Read the model definition and answer for the solid it produces. Units are mm, in the model's axes. Face numbers are marked on the shaded views. A direction names the side the tool comes from. Give positions to 0.01 mm unless a question says otherwise; leave off trailing zeros. Order: outer loops, then holes, each group sorted by start corner. A loop starts at its lowest first (then second) coordinate and runs counter-clockwise, first axis right, second up.
Item 1: Which of the six approach directions +Z, -Z, +X, -X, +Y, -Y give full straight-line access (tool end or side, diameter ignored) to the marked faces 1, 2, 3, 4 and 5?
Item 2: Given pin 1 Ø8 at (x, y) = (0, 8.5) entering from -Z; pin 2 Ø3 at (y, z) = (2, -9.5) entering from +X; pin 3 Ø12 at (y, z) = (2.5, 7.5) entering from +X; pin 4 Ø4 at (x, z) = (3.175, 6.35) entering from -Y, each flat-ended and moving along its own axis, determine where each tip first touches the part or whether it passes through.
Item 3: A cutting plane is placed at D-D (y = 9.75). Write down the section's boundary in (x, z) (3 decimals).
Item 4: Find the intervals of material crossed by line 1 along X through (y, z) = (8.75, 0); line 2 along X through (y, z) = (10.75, 0); line 3 along Y through (x, z) = (0, -5), in increasing order.
Item 5: The mould has two halves that part along Z. Classify the marked faces 6, 7 and 8: +Z half, -Z half, draft (parallel to the pull), parting line (faces both ways), or undercut.
Item 6: A cutting plane is placed at A-A (z = 0). State how many separate pieces and enclosed holes the cut face has, plus the area to 3 significant figures.
from build123d import *

# Parameters (mm, degrees)
SKETCH1_R               = 11.43
BOSS_EXTRUDE1_DEPTH     = 13.97
CUT_EXTRUDE1_DEPTH      = 5.08
CUT_EXTRUDE2_DEPTH      = 22.364706878
CUT_EXTRUDE2_DEPTH_BACK = 22.364706878
SKETCH3_R               = 2.286
FILLET1_R               = 1.27
SKETCH4_R               = 17.78
SKETCH4_R_2             = 11.43
BOSS_EXTRUDE2_DEPTH     = 6.35
CUT_EXTRUDE3_DEPTH      = 38.588567411
CUT_EXTRUDE3_DEPTH_BACK = 4.826
SKETCH5_R               = 4.064
SKETCH7_R               = 1.778
CUT_EXTRUDE4_DEPTH      = 29.764869198
CHAMFER1_SIZE           = 5.08
FILLET2_R               = 2.54
SKETCH9_R               = 2.032
CUT_EXTRUDE5_DEPTH      = 10.16


with BuildPart() as part:
    # Sketch1 → Boss-Extrude1 (new, symmetric)
    with BuildSketch(Plane(origin=(0, 0, 0), x_dir=(1, 0, 0), z_dir=(0, 1, 0))):
        with Locations(Location((0, 0, 0), (0, 0, 270))):
            Circle(SKETCH1_R)
    extrude(amount=BOSS_EXTRUDE1_DEPTH, both=True)

    # Sketch2 → Cut-Extrude1 (cut, symmetric)
    with BuildSketch(Plane(origin=(0, 0, 0), x_dir=(1, 0, 0), z_dir=(0, 1, 0))):
        with BuildLine():
            Line((10.980176456, 3.175), (0.790573729, 3.175))
            ThreePointArc((0.790573729, 3.175), (1.644174222, 7.956847789), (-1.908379573, 11.269560213))
            ThreePointArc((-1.908379573, 11.269560213), (-9.679362018, 6.079050167), (-10.980176456, -3.175))
            Line((-10.980176456, -3.175), (-0.790573729, -3.175))
            ThreePointArc((-0.790573729, -3.175), (-1.644174222, -7.956847789), (1.908379573, -11.269560213))
            ThreePointArc((1.908379573, -11.269560213), (8.730912854, -7.376724255), (11.43, 0))
            ThreePointArc((11.43, 0), (11.316985396, 1.603353222), (10.980176456, 3.175))
        make_face()
    extrude(amount=CUT_EXTRUDE1_DEPTH, both=True, mode=Mode.SUBTRACT)

    # Sketch3 → Cut-Extrude2 (cut, two sides: drawn at the far end of the back side and taken through both)
    with BuildSketch(Plane(origin=(0, 0, 0), x_dir=(1, 0, 0), z_dir=(0, 1, 0)).offset(-CUT_EXTRUDE2_DEPTH_BACK)):
        with Locations(Location((-3.175, 6.35, 0), (0, 0, 270))):
            Circle(SKETCH3_R)
        with Locations(Location((3.175, -6.35, 0), (0, 0, 270))):
            Circle(SKETCH3_R)
    extrude(amount=CUT_EXTRUDE2_DEPTH + CUT_EXTRUDE2_DEPTH_BACK, mode=Mode.SUBTRACT)

    # Fillet1
    # the kernel refuses this fillet: 1.27 mm, written as the material it takes off along each edge
    with BuildSketch(Plane(origin=(-0.790573729, 5.08, 3.175), x_dir=(-0.4705483235385416, 0, 0.8823742262867087), z_dir=(0, -1, 0))) as fillet1_piece_1:
        with BuildLine():
            CenterArc((2.104974221, 1.248277745), FILLET1_R, 151.930104711, 107.457603124)
            Line((0.984358954, 1.845874115), (0, 0))
            ThreePointArc((0, 0), (0.935544098, 0.086889022), (1.871088197, 0))
        make_face()
    extrude(amount=10.16, mode=Mode.SUBTRACT)
    with BuildSketch(Plane(origin=(-10.980176456, 5.08, 3.175), x_dir=(0.35895527903729396, 0, 0.9333547598053263), z_dir=(0, -1, 0))) as fillet1_piece_2:
        with BuildLine():
            CenterArc((1.847316222, -1.265342552), FILLET1_R, 85.09157022, 115.944479772)
            Line((0.661955677, -1.721215757), (0, 0))
            ThreePointArc((0, 0), (0.977990941, 0.041917031), (1.955981882, 0))
        make_face()
    extrude(amount=10.16, mode=Mode.SUBTRACT)
    with BuildSketch(Plane(origin=(-1.908379573, -5.08, -11.269560213), x_dir=(0.9998377506147018, 0, 0.018013118712026065), z_dir=(0, 1, 0))) as fillet1_piece_3:
        with BuildLine():
            CenterArc((3.987576413, -1.248150652), FILLET1_R, 79.35661856, 136.209501667)
            ThreePointArc((2.954501471, -1.986836082), (1.657014707, -0.726102119), (0, 0))
            ThreePointArc((0, 0), (2.111069866, 0.196644134), (4.222139731, 0))
        make_face()
    extrude(amount=10.16, mode=Mode.SUBTRACT)
    with BuildSketch(Plane(origin=(0.790573729, -5.08, -3.175), x_dir=(1, 0, 0), z_dir=(0, 1, 0))) as fillet1_piece_4:
        with BuildLine():
            CenterArc((2.0919402, 1.27), FILLET1_R, 162.542396876, 107.457603124)
            ThreePointArc((0.880437414, 1.651), (0.516887341, 0.784614516), (0, 0))
            Line((0, 0), (2.0919402, 0))
        make_face()
    extrude(amount=10.16, mode=Mode.SUBTRACT)
    with BuildSketch(Plane(origin=(10.980176456, -5.08, -3.175), x_dir=(-0.3589552790375579, 0, -0.9333547598052248), z_dir=(0, 1, 0))) as fillet1_piece_5:
        with BuildLine():
            CenterArc((1.847316222, 1.265342552), FILLET1_R, 158.963950007, 115.944479772)
            Line((0.661955677, 1.721215757), (0, 0))
            ThreePointArc((0, 0), (0.977990941, -0.041917031), (1.955981882, 0))
        make_face()
    extrude(amount=10.16, mode=Mode.SUBTRACT)
    with BuildSketch(Plane(origin=(1.908379573, 5.08, 11.269560213), x_dir=(-0.9998377506147016, 0, -0.018013118712031834), z_dir=(0, -1, 0))) as fillet1_piece_6:
        with BuildLine():
            CenterArc((3.987576413, 1.248150652), FILLET1_R, 144.433879773, 136.209501667)
            ThreePointArc((2.954501471, 1.986836082), (1.657014707, 0.726102119), (0, 0))
            ThreePointArc((0, 0), (2.111069866, -0.196644134), (4.222139731, 0))
        make_face()
    extrude(amount=10.16, mode=Mode.SUBTRACT)

    # Sketch4 → Boss-Extrude2 (add)
    with BuildSketch(Plane(origin=(0, 13.97, 0), x_dir=(1, 0, 0), z_dir=(0, 1, 0))):
        with Locations(Location((0, 0, 0), (0, 0, 270))):
            Circle(SKETCH4_R)
        with Locations(Location((0, 0, 0), (0, 0, 270))):
            Circle(SKETCH4_R_2, mode=Mode.SUBTRACT)
    boss_extrude2 = extrude(amount=-BOSS_EXTRUDE2_DEPTH)

    # Mirror1: Boss-Extrude2 across plane
    add(boss_extrude2.mirror(Plane.ZX))

    # Sketch5 → Cut-Extrude3 (cut, two sides: drawn at the far end of the back side and taken through both)
    with BuildSketch(Plane(origin=(0, 13.97, 0), x_dir=(1, 0, 0), z_dir=(0, 1, 0)).offset(-CUT_EXTRUDE3_DEPTH_BACK)):
        with Locations(Location((-3.175, 6.35, 0), (0, 0, 90))):
            Circle(SKETCH5_R)
        with Locations(Location((3.175, -6.35, 0), (0, 0, 90))):
            Circle(SKETCH5_R)
    extrude(amount=CUT_EXTRUDE3_DEPTH + CUT_EXTRUDE3_DEPTH_BACK, mode=Mode.SUBTRACT)

    # Sketch7 → Cut-Extrude4 (cut, through all)
    with BuildSketch(Plane(origin=(0, 0, 0), x_dir=(1, 0, 0), z_dir=(0, 1, 0))):
        with Locations(Location((-4.064, 0, 0), (0, 0, 270))):
            Circle(SKETCH7_R)
        with Locations(Location((4.064, 0, 0), (0, 0, 90))):
            Circle(SKETCH7_R)
    extrude(amount=CUT_EXTRUDE4_DEPTH, mode=Mode.SUBTRACT)

    # Chamfer1
    chamfer1_edges = [part.edges().sort_by_distance(p)[0] for p in [
        (0, 7.62, -17.78),
        (0, -7.62, -17.78),
    ]]
    chamfer(chamfer1_edges, length=CHAMFER1_SIZE)

    # Fillet2
    # the kernel refuses this fillet: 2.54 mm, written as the material it adds along each edge
    with BuildSketch(Plane(origin=(0, 7.62, 0), x_dir=(0, 0, 1), z_dir=(-1, 0, 0))) as fillet2_piece_1:
        with BuildLine():
            CenterArc((13.97, -2.199704526), FILLET2_R, 120, 60)
            Line((12.7, 0), (12.6746, 0.043994091))
            ThreePointArc((12.6746, 0.043994091), (12.065, 0.0508), (11.43, 0.0508))
            Line((11.43, 0.0508), (11.3792, 0))
            Line((11.3792, 0), (11.3792, -2.199704526))
            Line((11.3792, -2.199704526), (11.43, -2.199704526))
        make_face()
    revolve(axis=Axis((0, 7.62, 0), (0, 1, 0)))
    with BuildSketch(Plane(origin=(0, -7.62, 0), x_dir=(0, 0, 1), z_dir=(-1, 0, 0))) as fillet2_piece_2:
        with BuildLine():
            CenterArc((13.97, 2.199704526), FILLET2_R, 180, 60)
            Line((11.43, 2.199704526), (11.3792, 2.199704526))
            Line((11.3792, 2.199704526), (11.3792, 0))
            Line((11.3792, 0), (11.43, -0.0508))
            ThreePointArc((11.43, -0.0508), (12.065, -0.0508), (12.6746, -0.043994091))
            Line((12.6746, -0.043994091), (12.7, 0))
        make_face()
    revolve(axis=Axis((0, -7.62, 0), (0, 1, 0)))

    # Sketch9 → Cut-Extrude5 (cut)
    with BuildSketch(Plane.XZ.offset(13.97)):
        with Locations(Location((0, 0, 0), (0, 0, 270))):
            Circle(SKETCH9_R)
    extrude(amount=-CUT_EXTRUDE5_DEPTH, mode=Mode.SUBTRACT)


solid = part.part
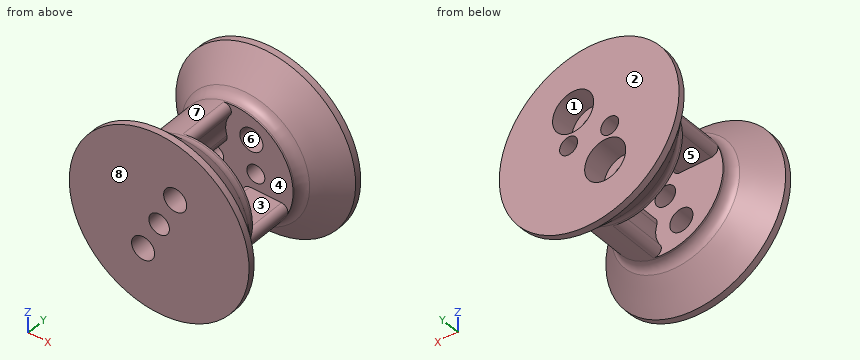
Response values:
1. face 1: +Y
1. face 2: +Z, -Z, +X, -X, +Y
1. face 3: +Z, +X, -X
1. face 4: none
1. face 5: -Z, +X, -X
2. pin 1: stops at z = -17.58
2. pin 2: stops at x = 8.16
2. pin 3: stops at x = 12.05
2. pin 4: passes through
3. outline: circle Ø29.66 at (0, 0); hole circle Ø8.128 at (-3.175, -6.35); hole circle Ø3.556 at (-4.064, 0); hole circle Ø8.128 at (3.175, 6.35); hole circle Ø3.556 at (4.064, 0)
4. line 1: x = -13.83 to -5.84, -2.29 to 2.29, 5.84 to 13.83
4. line 2: x = -15.83 to -5.84, -2.29 to 2.29, 5.84 to 15.83
4. line 3: y = -13.97 to -5.08, 5.08 to 9.14
5. face 6: undercut
5. face 7: parting line
5. face 8: draft
6. separate pieces: 5
6. enclosed holes: 0
6. area: 420 mm2
